Geometry: final body of the model. Coordinates: model frame, mm. Face numbers are marked on the shaded views. A direction names the side the tool comes from. Round coordinates to 2 decimals unless told otherwise and drop trailing zeros. Order: outer loops, then holes, each group sorted by start corner. A loop starts at its lowest first (then second) coordinate and runs counter-clockwise, first axis right, second up. Notation, with made-up numbers: M 50.25,11.25 L 60.25,11.25 A31 cw 60.25,41.25 Z; hole C 68,22 d11. An arc over 180 degrees is marked long. Return JSON: item names as keys, results as strings. Group by question number.
Q1. Cut plane A-A on x = 158. Output: boundary loops of the cut face in (y, z), and give its area (3 significant figures).
Q2. Access query for the marked faces 1 and 2. Directions: +Z, -Z, +X, -X, +Y, -Y. A direction counts if a zero-diameter tool reaches every point of the face in a straight line with its end or side. Return the directions, or none.
Q3. Contact query for flat-ended pins moving along their axis: pin 1 (2.5 mm diameter, centred on y = -2, z = 9.5, fed in from +X); pin 2 (4.5 mm diameter, centred on x = 155.5, y = 3, fed in from +Z); pin 3 (8 mm diameter, centred on x = 98.5, z = 9.5, fed in from -Y); pin 4 (8 mm diameter, centred on x = 114.5, z = 12.5, fed in from -Y). Output: stop coordinate, or through.
Q4. Ray query, probe 1 along Y at (x, z) = (158, 6); probe 2 along Y at (x, z) = (158, 14.65); probe 3 along Y at (x, z) = (8, 13.75). Return the intervals inside material, ascending.
Q5. Cut plane B-B on z = 3.75. Count the separate pieces of the cut face and the enclosed holes in it, and give its area (3 significant figures).
Q6. Cut plane C-C on x = 49. Output: boundary loops of the cut face in (y, z), and give its area (3 significant figures).
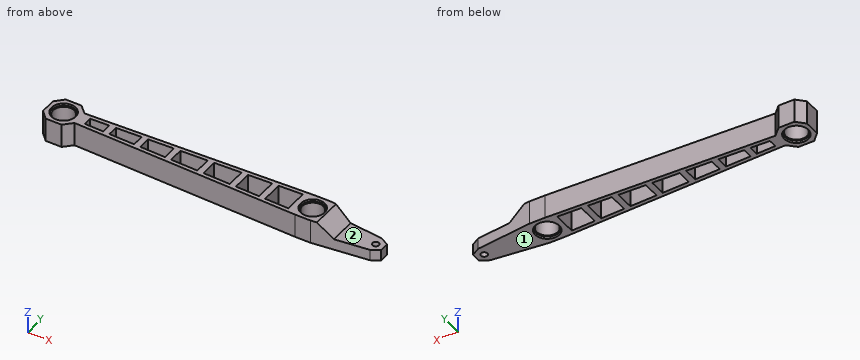
```python
from build123d import *

# Parameters (mm, degrees)
SKETCH_1_R          = 6.65
SKETCH_1_R_2        = 2.05
EXTRUDE_1_DEPTH     = 15
CUT_EXTRUDE_1_DEPTH = 205.728298873
SKETCH_3_R          = 7.65
CUT_EXTRUDE_2_DEPTH = 1.5
CUT_EXTRUDE_START   = -1.5
SKETCH_4_R          = 7.65
CUT_EXTRUDE_3_DEPTH = 1.5


with BuildPart() as part:
    # 草图1 → 凸台-拉伸1 (new body)
    with BuildSketch(Plane.XY):
        Polygon((198, 6), (203.196152423, 3), (203.196152423, -3), (198, -6), (163, -10), (153, -10), (10.101020514, -5), (5, -10), (-5, -10), (-9.898979486, -5), (-9.898979486, 5), (-5, 10), (5, 10), (10.101020514, 5), (153, 10), (163, 10), align=None)
        Circle(SKETCH_1_R, mode=Mode.SUBTRACT)
        with Locations((198, 0)):
            Circle(SKETCH_1_R_2, mode=Mode.SUBTRACT)
        with Locations((158, 0)):
            Circle(SKETCH_1_R, mode=Mode.SUBTRACT)
        Polygon((15.101020514, -2.67341888), (15.101020514, 2.67341888), (27.101020514, 3.093295916), (27.101020514, -3.093295916), align=None, mode=Mode.SUBTRACT)
        Polygon((31.101020514, -3.233254928), (31.101020514, 3.233254928), (47.101020514, 3.793090977), (47.101020514, -3.793090977), align=None, mode=Mode.SUBTRACT)
        Polygon((51.101020514, -3.933049989), (51.101020514, 3.933049989), (67.101020514, 4.492886037), (67.101020514, -4.492886037), align=None, mode=Mode.SUBTRACT)
        Polygon((71.101020514, 4.632845049), (88.101020514, 5.227670851), (88.101020514, -5.227670851), (71.101020514, -4.632845049), align=None, mode=Mode.SUBTRACT)
        Polygon((109.101020514, 5.962455664), (109.101020514, -5.962455664), (92.101020514, -5.367629863), (92.101020514, 5.367629863), align=None, mode=Mode.SUBTRACT)
        Polygon((113.101020514, -6.102414676), (128.101020514, -6.627260972), (128.101020514, 6.627260972), (113.101020514, 6.102414676), align=None, mode=Mode.SUBTRACT)
        Polygon((147.101020514, -7.292066279), (147.101020514, 7.292066279), (132.101020514, 6.767219984), (132.101020514, -6.767219984), align=None, mode=Mode.SUBTRACT)
    extrude(amount=EXTRUDE_1_DEPTH)

    # 草图2 → 切除-拉伸1 (cut, through all)
    with BuildSketch(Plane.XZ.offset(10)):
        Polygon((166.7, 15), (176.696152423, 7), (203.196152423, 7), (203.196152423, 15), align=None)
    extrude(amount=-CUT_EXTRUDE_1_DEPTH, mode=Mode.SUBTRACT)

    # 草图3 → 切除-拉伸2 (cut)
    with BuildSketch(Plane.XY.offset(15)):
        Circle(SKETCH_3_R)
        with Locations((158, 0)):
            Circle(SKETCH_3_R)
    extrude(amount=-CUT_EXTRUDE_2_DEPTH, mode=Mode.SUBTRACT)

    # 草图4 → 切除-拉伸3 (cut)
    with BuildSketch(Plane(origin=(0, 0, 0), x_dir=(-1, 0, 0), z_dir=(0, 0, -1)).offset(CUT_EXTRUDE_START)):
        with Locations(Location((-158, 0, 0), (0, 0, 180))):
            Circle(SKETCH_4_R)
        with Locations(Location((0, 0, 0), (0, 0, 180))):
            Circle(SKETCH_4_R)
    extrude(amount=CUT_EXTRUDE_3_DEPTH, mode=Mode.SUBTRACT)


solid = part.part
```
Result sheet:
{
 "1": {"outline": "M -10,0 L -7.65,0 L -7.65,1.5 L -6.65,1.5 L -6.65,13.5 L -7.65,13.5 L -7.65,15 L -10,15 Z; M 6.65,1.5 L 7.65,1.5 L 7.65,0 L 10,0 L 10,15 L 7.65,15 L 7.65,13.5 L 6.65,13.5 Z", "area": "94.5 mm²"},
 "2": {"face 1": "-Z, +X, -X, +Y, -Y", "face 2": "+Z, +X, +Y, -Y"},
 "3": {"pin 1": "stops at x = 175.13", "pin 2": "passes through", "pin 3": "stops at y = -8.23", "pin 4": "stops at y = -8.79"},
 "4": {"probe 1": "y = -10 to -6.65, 6.65 to 10", "probe 2": "y = -10 to -7.65, 7.65 to 10", "probe 3": "y = -7.06 to 7.06"},
 "5": {"separate pieces": "1", "enclosed holes": "10", "area": "1,930 mm²"},
 "6": {"outline": "M -6.36,0 L 6.36,0 L 6.36,15 L -6.36,15 Z", "area": "191 mm²"}
}
